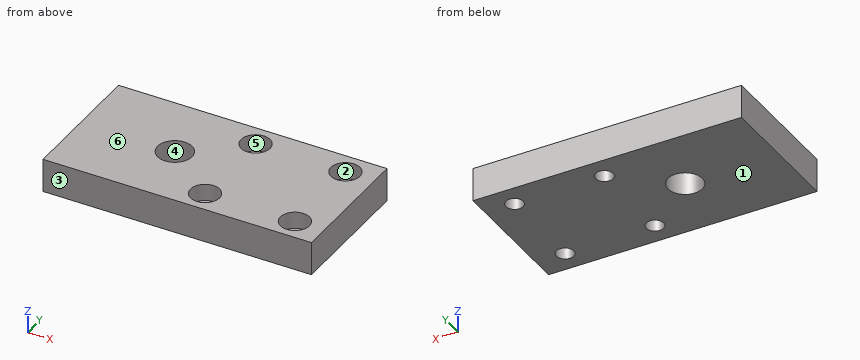
from build123d import *

# Parameters (mm, degrees)
CROQUIS1_W                                           = 101.6
CROQUIS1_H                                           = 50.8
CROQUIS1_R                                           = 6.5
SALIENTE_EXTRUIR1_DEPTH                              = 6.35
REFRENTADO_PARA_TORNILLO_CON_CABEZA_HUEC_D           = 6.6
REFRENTADO_PARA_TORNILLO_CON_CABEZA_HUEC_CBORE_D     = 11
REFRENTADO_PARA_TORNILLO_CON_CABEZA_HUEC_CBORE_DEPTH = 6.4


with BuildPart() as part:
    # Croquis1 → Saliente-Extruir1 (new, symmetric)
    with BuildSketch(Plane.XY):
        Rectangle(CROQUIS1_W, CROQUIS1_H)
        with Locations((-15.2, 0)):
            Circle(CROQUIS1_R, mode=Mode.SUBTRACT)
    extrude(amount=SALIENTE_EXTRUIR1_DEPTH, both=True)

    # Refrentado para tornillo con cabeza hueca de M61 (through all)
    with Locations(Plane.XY.offset(6.35)):
        with Locations((5.8, 17), (39.8, 17), (39.8, -17), (5.8, -17)):
            CounterBoreHole(REFRENTADO_PARA_TORNILLO_CON_CABEZA_HUEC_D / 2, REFRENTADO_PARA_TORNILLO_CON_CABEZA_HUEC_CBORE_D / 2, REFRENTADO_PARA_TORNILLO_CON_CABEZA_HUEC_CBORE_DEPTH)


solid = part.part
Here's how the part is built. I have some questions about the finished solid (model axes, mm). Face numbers are marked on the shaded views. A direction names the side the tool comes from. Coordinates: 2 decimals unless noted, no trailing zeros. Order: outer loops, then holes, each group sorted by start corner. A loop starts at its lowest first (then second) coordinate and runs counter-clockwise, first axis right, second up. Notation, with made-up numbers: M 55,89 L 69,89 A18 ccw 69,110 Z; hole C 71,30 d7. An arc over 180 degrees is marked long. Answer as CSV lines item,"result". Start each with the question number.
1. On a 3-axis mill with a long thin cutter (end or side, diameter ignored), from which of +Z, -Z, +X, -X, +Y, -Y can I reach the whole of each face in a straight line? I mean the marked faces 5 and 6. Say none if no direction works.
2. I want a section at B-B, the plane z = -3.5. Write out the boundary of the cut face in (x, y).
3. I want a section at A-A, the plane y = -17. Write out the boundary of the cut face in (x, z), and give its area (3 significant figures).
4. I need wall thicknesses on line 1 (Y direction, x = 39.8, z = 2); line 2 (Y direction, x = 39.8, z = -2.5); line 3 (Y direction, x = -15.5, z = 2.25). Which ranges of each line are inside material? Lowest first, please. Write a range as [from, to].
5. I want a section at D-D, the plane y = -2. Write out the boundary of the cut face in (x, z).
6. For pin 1 (5.5 mm diameter, centred on x = 5, y = 15, fed in from +Z), with a flat end and sliding along its axis, tell me the tip position at first contact or that it passes through.
7. We'd pull the mould along Y, two halves only. Please class the marked faces 1, 2, 3 and 4: released by +Y, released by -Y, zero draft, split by the parting line, or undercut.
8. I want a section at C-C, the plane x = 5.8. Write out the boundary of the cut face in (y, z), and give its area (3 significant figures).
Recorded:
1,face 5,"+Z"
1,face 6,"+Z, +X, -X, +Y, -Y"
2,outline,"M -50.8,-25.4 L 50.8,-25.4 L 50.8,25.4 L -50.8,25.4 Z; hole C -15.2,0 d13; hole C 5.8,-17 d6.6; hole C 5.8,17 d6.6; hole C 39.8,-17 d6.6; hole C 39.8,17 d6.6"
3,outline,"M -50.8,-6.35 L 2.5,-6.35 L 2.5,-0.05 L 0.3,-0.05 L 0.3,6.35 L -50.8,6.35 Z; M 9.1,-6.35 L 36.5,-6.35 L 36.5,-0.05 L 34.3,-0.05 L 34.3,6.35 L 11.3,6.35 L 11.3,-0.05 L 9.1,-0.05 Z; M 43.1,-6.35 L 50.8,-6.35 L 50.8,6.35 L 45.3,6.35 L 45.3,-0.05 L 43.1,-0.05 Z"
3,area,"1,070 mm2"
4,line 1,"y = [-25.4, -22.5], [-11.5, 11.5], [22.5, 25.4]"
4,line 2,"y = [-25.4, -20.3], [-13.7, 13.7], [20.3, 25.4]"
4,line 3,"y = [-25.4, -6.49], [6.49, 25.4]"
5,outline,"M -50.8,-6.35 L -21.38,-6.35 L -21.38,6.35 L -50.8,6.35 Z; M -9.02,-6.35 L 50.8,-6.35 L 50.8,6.35 L -9.02,6.35 Z"
6,pin 1,"stops at z = -0.05"
7,face 1,"zero draft"
7,face 2,"undercut"
7,face 3,"released by -Y"
7,face 4,"undercut"
8,outline,"M -25.4,-6.35 L -20.3,-6.35 L -20.3,-0.05 L -22.5,-0.05 L -22.5,6.35 L -25.4,6.35 Z; M -13.7,-6.35 L 13.7,-6.35 L 13.7,-0.05 L 11.5,-0.05 L 11.5,6.35 L -11.5,6.35 L -11.5,-0.05 L -13.7,-0.05 Z; M 20.3,-6.35 L 25.4,-6.35 L 25.4,6.35 L 22.5,6.35 L 22.5,-0.05 L 20.3,-0.05 Z"
8,area,"421 mm2"
